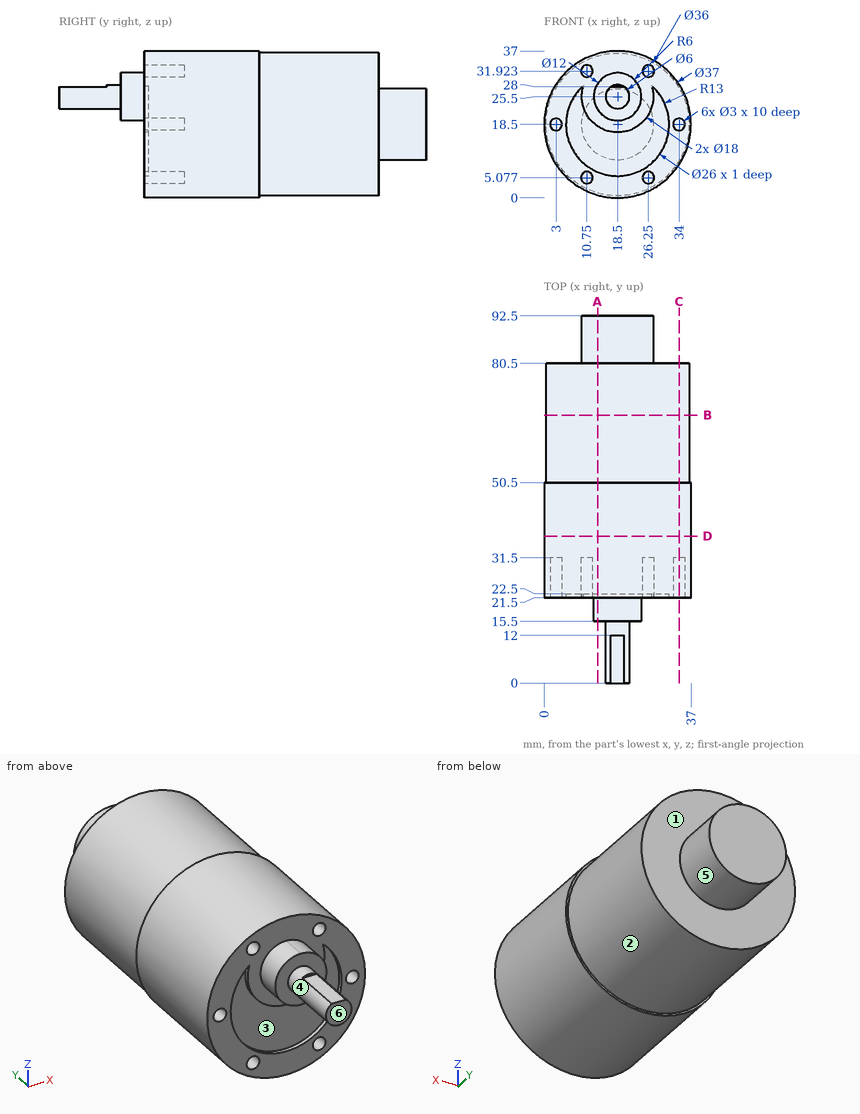
Design review of the part shown in the three views and the two pictorial views. Dimensions are in mm from the part's minimum x, y and z. A direction names the side the tool comes from. Give positions to 0.01 mm unless a question says otherwise; leave off trailing zeros. Loops run counter-clockwise (first coordinate to the right, second up) from the corner with the lowest first, then second, coordinate; pieces in that order, holes last. Notation, with made-up numbers: (76.5, 43.25) - (135.5, 43.25) arc R10 cw to (135.5, 49.25) - close; hole circle Ø8 at (23.5, 14.5). An arc over 180 degrees is marked (long way). Write item = value, one per line.
1) To check wall thickness, follow line 1 (Z direction, x = 26, y = 24) (1 decimal); line 2 (Z direction, x = 18, y = 22); line 3 (X direction, y = 27, z = 18) (1 decimal). State the ranges of each line that lie inside material, in increasing order.
Result sheet:
line_1 = 1.6 to 3.6, 6.6 to 30.4, 33.4 to 35.4
line_2 = 0.01 to 5.51, 16.51 to 36.99
line_3 = 0 to 1.6, 4.4 to 32.6, 35.4 to 37
2) Tool access review of the marked faces 4, 5 and 6: name each direction out of +Z, -Z, +X, -X, +Y, -Y from which nothing blocks a thin tool from reaching the whole face with its end or side.
Result sheet:
face_4 = -Y
face_5 = +Y
face_6 = +Z, -Z, +X, -X, -Y
3) Clearance check with flat-ended pins moving along their axes: pin 1 Ø5 at (x, z) = (10.75, 31.92) entering from +Y; pin 2 Ø5 at (x, y) = (16, 9.5) entering from -Z; pin 3 Ø1.5 at (x, y) = (14.5, 15.5) entering from -Z. State where each tip first meets the part, or that it passes through.
Result sheet:
pin_1 = 80.5
pin_2 = 22.5
pin_3 = 20.46
4) Take a section at C-C on x = 34. State the section outline as (y, z) points.
Result sheet:
outline = (21.5, 8.4) - (50.5, 8.4) - (50.5, 9.35) - (80.5, 9.35) - (80.5, 27.65) - (50.5, 27.65) - (50.5, 28.6) - (21.5, 28.6) - (21.5, 20) - (31.5, 20) - (31.5, 17) - (21.5, 17) - close
5) Take a section at D-D on y = 37. State the section outline as (x, z) points.
Result sheet:
outline = circle Ø37 at (18.5, 18.5)
6) Take a section at A-A on x = 13.5. State the section outline as (y, z) points, and give its area (3 significant figures).
Result sheet:
outline = (15.5, 22.18) - (21.5, 22.18) - (21.5, 18.02) - (22.5, 18.02) - (22.5, 6.5) - (21.5, 6.5) - (21.5, 0.69) - (50.5, 0.69) - (50.5, 1.21) - (80.5, 1.21) - (80.5, 11.02) - (92.5, 11.02) - (92.5, 25.98) - (80.5, 25.98) - (80.5, 35.79) - (50.5, 35.79) - (50.5, 36.31) - (21.5, 36.31) - (21.5, 28.82) - (15.5, 28.82) - close
area = 2,280 mm2
7) Take a section at B-B on y = 67.5. State the section outline as (x, z) points.
Result sheet:
outline = circle Ø36 at (18.5, 18.5)
8) Draft analysis for pull direction X (two halves, no side actions). For the marked faces 1, 2 and 3, state which applies: +X half, -X half, draft (parallel to the pull), parting line (faces both ways), or undercut.
Result sheet:
face_1 = draft
face_2 = parting line
face_3 = undercut
